Input: part model. Units: mm. Frame: model coordinates. A direction names the side the tool comes from. Round coordinates to 2 decimals unless told otherwise and drop trailing zeros. Loops run counter-clockwise (first coordinate to the right, second up) from the corner with the lowest first, then second, coordinate; pieces in that order, holes last.
1) Ray query, line 1 along Y through (x, z) = (0, 2); line 2 along Y through (x, z) = (0, 0); line 3 along Y through (x, z) = (13.5, -4). Return the intervals inside material, ascending.
2) Draft query along Y for faces 1 (the face through (3.6, 10, 7)), 2 (the face through (-15, -7, -6.75)). Return one class per face: pulls with the +Y half, pulls with the -Y half, needs draft (parallel to the pull), parting line crosses it, or undercut.
3) First-contact query: pin 1 (1.5 mm diameter, centred on y = 18, z = 1, fed in from -X); pin 2 (7.5 mm diameter, centred on x = -17.5, y = 17.5, fed in from +Z); pin 3 (14.5 mm diameter, centred on x = 17.5, y = -17.5, fed in from -Z); pin 4 (1 mm diameter, centred on x = 3, z = -4, fed in from -Y). Flat tips, straight axial feed; report the tip coordinate or a pass-through.
4) Section C-C, the plane y = 24.75. Return loops of the section in (x, z).
5) Section B-B, the plane x = 0. State how many separate pieces and enclosed holes the cut face has, and give its area (3 significant figures).
6) Section A-A, the plane z = 6.5. Return loops of the section in (x, y).
7) Access query for faces 3 (the face through (-0.293, 13.545, 1.454)), 4 (the face through (18.5, -21.99, -5.27)), 5 (the face through (-0.079, 14.913, 6.778)). Directions: +Z, -Z, +X, -X, +Y, -Y. A direction counts if a zero-diameter tool reaches every point of the face in a straight line with its end or side. Return the directions, or none.
from build123d import *
from build123d.topology import SkipClean

# Parameters (mm, degrees)
SKETCH1_R               = 34.1
BOSS_EXTRUDE1_DEPTH     = 1.75
SKETCH4_R               = 28.5
BOSS_EXTRUDE2_DEPTH     = 2
SKETCH5_R               = 34.1
SKETCH5_R_2             = 16.25
BOSS_EXTRUDE3_DEPTH     = 5
CUT_EXTRUDE2_DEPTH      = 49.968050809
CUT_EXTRUDE2_DEPTH_BACK = 49.968050809
SKETCH3_R               = 2.25
CUT_EXTRUDE1_DEPTH      = 49.968050809
CUT_EXTRUDE1_DEPTH_BACK = 49.968050809
SKETCH2_R               = 7.25
SKETCH6_R               = 2.25
CUT_EXTRUDE3_DEPTH      = 50.354533733
CIRPATTERN1_COUNT       = 8
SKETCH7_R               = 20.5
SKETCH7_R_2             = 2.25
SKETCH7_R_3             = 7.25
BOSS_EXTRUDE4_DEPTH     = 5
BOSS_EXTRUDE5_START     = 2
SKETCH8_R               = 34.1
SKETCH8_R_2             = 28.5
BOSS_EXTRUDE5_DEPTH     = 2
SKETCH10_R              = 34.1
SKETCH10_R_2            = 20.5
CUT_EXTRUDE4_DEPTH      = 2
CUT_EXTRUDE5_DEPTH      = 4
SKETCH12_R              = 4.6
CUT_EXTRUDE6_DEPTH      = 3
FILLET2_R               = 1


with BuildPart() as part:
    # Sketch1 → Boss-Extrude1 (new, symmetric)
    with BuildSketch(Plane.XY):
        Circle(SKETCH1_R)
    extrude(amount=BOSS_EXTRUDE1_DEPTH, both=True)

    # Sketch4 → Boss-Extrude2 (add)
    with BuildSketch(Plane.XY.offset(1.75)):
        Circle(SKETCH4_R)
    extrude(amount=BOSS_EXTRUDE2_DEPTH)

    # Sketch5 → Boss-Extrude3 (add)
    with BuildSketch(Plane(origin=(0, 0, -1.75), x_dir=(-1, 0, 0), z_dir=(0, 0, -1))):
        Circle(SKETCH5_R)
        Circle(SKETCH5_R_2, mode=Mode.SUBTRACT)
    extrude(amount=BOSS_EXTRUDE3_DEPTH)

    # Sketch3 → Cut-Extrude2 (cut, two sides: drawn at the far end of the back side and taken through both)
    with BuildSketch(Plane.XY.offset(1.75).offset(-CUT_EXTRUDE2_DEPTH_BACK)):
        with Locations((0, 11.3137085)):
            Circle(SKETCH3_R)
        with Locations((11.3137085, 0)):
            Circle(SKETCH3_R)
        with Locations((0, -11.3137085)):
            Circle(SKETCH3_R)
        with Locations((-11.3137085, 0)):
            Circle(SKETCH3_R)
    extrude(amount=CUT_EXTRUDE2_DEPTH + CUT_EXTRUDE2_DEPTH_BACK, mode=Mode.SUBTRACT)

    # Sketch2 → Cut-Extrude1 (cut, two sides: drawn at the far end of the back side and taken through both)
    with BuildSketch(Plane.XY.offset(1.75).offset(-CUT_EXTRUDE1_DEPTH_BACK)):
        Circle(SKETCH2_R)
    extrude(amount=CUT_EXTRUDE1_DEPTH + CUT_EXTRUDE1_DEPTH_BACK, mode=Mode.SUBTRACT)

    # Sketch6 → Cut-Extrude3 (cut, symmetric)
    with BuildSketch(Plane.XY.offset(3.75)):
        with Locations((0, 24.75)):
            Circle(SKETCH6_R)
    cut_extrude3 = extrude(amount=CUT_EXTRUDE3_DEPTH, both=True, mode=Mode.SUBTRACT)

    # CirPattern1: Cut-Extrude3 ×8 about axis
    cirpattern1_axis = Axis((0, 0, 0), (0, 0, 1))
    for i in range(1, CIRPATTERN1_COUNT):
        add(cut_extrude3.rotate(cirpattern1_axis, i * 360 / CIRPATTERN1_COUNT), mode=Mode.SUBTRACT)

    # Sketch7 → Boss-Extrude4 (add)
    with BuildSketch(Plane.XY.offset(3.75)):
        Circle(SKETCH7_R)
        with Locations((0, -11.3137085)):
            Circle(SKETCH7_R_2, mode=Mode.SUBTRACT)
        with Locations((11.3137085, 0)):
            Circle(SKETCH7_R_2, mode=Mode.SUBTRACT)
        with Locations((0, 11.3137085)):
            Circle(SKETCH7_R_2, mode=Mode.SUBTRACT)
        with Locations((-11.3137085, 0)):
            Circle(SKETCH7_R_2, mode=Mode.SUBTRACT)
        Circle(SKETCH7_R_3, mode=Mode.SUBTRACT)
    extrude(amount=BOSS_EXTRUDE4_DEPTH)

    # Sketch8 → Boss-Extrude5 (add)
    with SkipClean():  # the faces are left unmerged after this step: merging them gives an invalid solid
        with BuildSketch(Plane.XY.offset(1.75).offset(BOSS_EXTRUDE5_START)):
            with Locations(Location((0, 0, 0), (0, 0, 180))):
                Circle(SKETCH8_R)
            Circle(SKETCH8_R_2, mode=Mode.SUBTRACT)
        extrude(amount=-BOSS_EXTRUDE5_DEPTH)

    # Sketch10 → Cut-Extrude4 (cut)
    with BuildSketch(Plane.XY.offset(3.75)):
        with Locations(Location((0, 0, 0), (0, 0, 180))):
            Circle(SKETCH10_R)
        Circle(SKETCH10_R_2, mode=Mode.SUBTRACT)
    extrude(amount=-CUT_EXTRUDE4_DEPTH, mode=Mode.SUBTRACT)

    # Sketch11 → Cut-Extrude5 (cut)
    with BuildSketch(Plane.XY.offset(8.75)):
        with BuildLine():
            Line((-11.3137085, 3.6), (-8.248636251, 3.6))
            ThreePointArc((-8.248636251, 3.6), (-6.363961031, 6.363961031), (-3.6, 8.248636251))
            Line((-3.6, 8.248636251), (-3.6, 11.3137085))
            ThreePointArc((-3.6, 11.3137085), (0, 14.9137085), (3.6, 11.3137085))
            Line((3.6, 11.3137085), (3.6, 8.248636251))
            ThreePointArc((3.6, 8.248636251), (6.363961031, 6.363961031), (8.248636251, 3.6))
            Line((8.248636251, 3.6), (11.3137085, 3.6))
            ThreePointArc((11.3137085, 3.6), (14.9137085, 0), (11.3137085, -3.6))
            Line((11.3137085, -3.6), (8.248636251, -3.6))
            ThreePointArc((8.248636251, -3.6), (6.363961031, -6.363961031), (3.6, -8.248636251))
            Line((3.6, -8.248636251), (3.6, -11.3137085))
            ThreePointArc((3.6, -11.3137085), (0, -14.9137085), (-3.6, -11.3137085))
            Line((-3.6, -11.3137085), (-3.6, -8.248636251))
            ThreePointArc((-3.6, -8.248636251), (-6.363961031, -6.363961031), (-8.248636251, -3.6))
            Line((-8.248636251, -3.6), (-11.3137085, -3.6))
            ThreePointArc((-11.3137085, -3.6), (-14.9137085, 0), (-11.3137085, 3.6))
        make_face()
    extrude(amount=-CUT_EXTRUDE5_DEPTH, mode=Mode.SUBTRACT)

    # Sketch12 → Cut-Extrude6 (cut)
    with BuildSketch(Plane(origin=(0, 0, -6.75), x_dir=(-1, 0, 0), z_dir=(0, 0, -1))):
        with Locations((0, 24.75)):
            Circle(SKETCH12_R)
        with Locations((17.500892834, 17.500892834)):
            Circle(SKETCH12_R)
        with Locations((24.75, 0)):
            Circle(SKETCH12_R)
        with Locations((17.500892834, -17.500892834)):
            Circle(SKETCH12_R)
        with Locations((0, -24.75)):
            Circle(SKETCH12_R)
        with Locations((-17.500892834, -17.500892834)):
            Circle(SKETCH12_R)
        with Locations((-24.75, 0)):
            Circle(SKETCH12_R)
        with Locations((-17.500892834, 17.500892834)):
            Circle(SKETCH12_R)
    extrude(amount=-CUT_EXTRUDE6_DEPTH, mode=Mode.SUBTRACT)

    # Fillet2
    fillet2_edges = [part.edges().sort_by_distance(p)[0] for p in [
        (-20.5, 0, 8.75),
    ]]
    fillet(fillet2_edges, radius=FILLET2_R)


solid = part.part
Final values:
1. line 1: y = -20.5 to -13.56, -9.06 to -7.25, 7.25 to 9.06, 13.56 to 20.5
1. line 2: y = -34.1 to -27, -22.5 to -13.56, -9.06 to -7.25, 7.25 to 9.06, 13.56 to 22.5, 27 to 34.1
1. line 3: y = -31.31 to -19.77, -15.23 to -9.05, 9.05 to 15.23, 19.77 to 31.31
2. face 1: undercut
2. face 2: needs draft
3. pin 1: stops at x = -29.42
3. pin 2: stops at z = 1.75
3. pin 3: stops at z = -6.75
3. pin 4: stops at y = -34.01
4. outline: (-23.46, -6.75) - (-4.6, -6.75) - (-4.6, -3.75) - (-2.25, -3.75) - (-2.25, 1.75) - (-23.46, 1.75) - close; (2.25, -3.75) - (4.6, -3.75) - (4.6, -6.75) - (23.46, -6.75) - (23.46, 1.75) - (2.25, 1.75) - close
5. separate pieces: 6
5. enclosed holes: 0
5. area: 327 mm2
6. outline: circle Ø41 at (0, 0); hole (-11.31, -3.6) - (-8.25, -3.6) arc R9 ccw to (-3.6, -8.25) - (-3.6, -11.31) arc R3.6 ccw to (3.6, -11.31) - (3.6, -8.25) arc R9 ccw to (8.25, -3.6) - (11.31, -3.6) arc R3.6 ccw to (11.31, 3.6) - (8.25, 3.6) arc R9 ccw to (3.6, 8.25) - (3.6, 11.31) arc R3.6 ccw to (-3.6, 11.31) - (-3.6, 8.25) arc R9 ccw to (-8.25, 3.6) - (-11.31, 3.6) arc R3.6 ccw to start
7. face 3: +Z, -Z
7. face 4: -Z
7. face 5: +Z
